Source: CAD feature listing. Evaluate the final solid. Frame: model axes, mm. Round coordinates to 2 decimals unless told otherwise and drop trailing zeros. Write each loop counter-clockwise with the first axis right and the second up, starting at its lowest first coordinate (ties: lowest second). Pieces come first, ordered by that corner, then holes. Notation, with made-up numbers: M -26,-12 L -13,-12 A26 cw -13,11 Z; hole C -31.75,63.5 d7. An arc over 180 degrees is marked long. Answer in a Markdown table with one row per item. Add a question column.
Item 1: Cut plane B-B on z = -34.75. Give the number of separate pieces and of enclosed holes in the cut face, and give its area (3 significant figures).
Item 2: Cut plane A-A on x = 276. Return loops of the section in (y, z).
Item 3: Material intervals for probe 1 along X at (y, z) = (53.75, -211.5); probe 2 along X at (y, z) = (56.25, -34.75); probe 3 along X at (y, z) = (42, -184), sorted ascending.
Item 4: Contact query for flat-ended pins moving along their axis: pin 1 (5.5 mm diameter, centred on x = 23.5, z = -34.5, fed in from +Y); pin 2 (4.5 mm diameter, centred on x = 261, z = -211.5, fed in from +Y). Output: stop coordinate, or through.
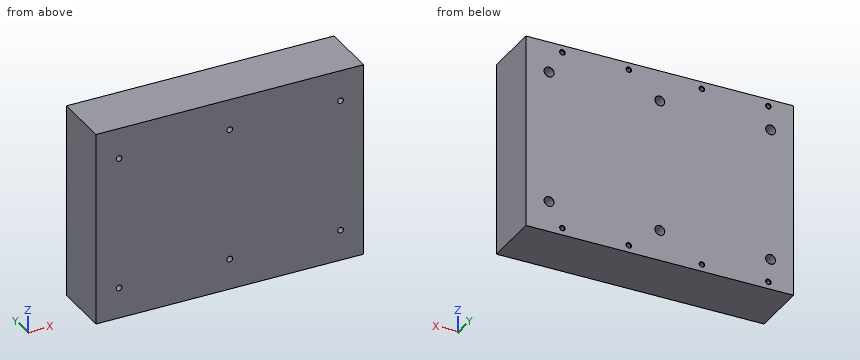
from build123d import *

# Parameters (mm, degrees)
SKETCH1_W                       = 302
SKETCH1_H                       = 219.5
BOSS_EXTRUDE1_DEPTH             = 64.4
M6X1_0_TAPPED_HOLE1_D           = 5
M6X1_0_TAPPED_HOLE1_DEPTH       = 16
M6X1_0_TAPPED_HOLE1_CSINK_D     = 6.2
M6X1_0_TAPPED_HOLE1_CSINK_ANGLE = 90
M6X1_0_TAPPED_HOLE1_TIP         = 1.502151548
CBORE_FOR_M6_SHCS1_AT_2_COUNT   = 2
CBORE_FOR_M6_SHCS1_AT_2_PITCH   = 150
CBORE_FOR_M6_SHCS1_AT_3_COUNT   = 2
CBORE_FOR_M6_SHCS1_AT_3_PITCH   = 195.256241898
CBORE_FOR_M6_SHCS1_AT_4_COUNT   = 2
CBORE_FOR_M6_SHCS1_AT_4_PITCH   = 125
CBORE_FOR_M6_SHCS1_AT_5_COUNT   = 2
CBORE_FOR_M6_SHCS1_AT_5_PITCH   = 250
CBORE_FOR_M6_SHCS1_AT_6_COUNT   = 2
CBORE_FOR_M6_SHCS1_AT_6_PITCH   = 291.547594742


with BuildPart() as part:
    # Sketch1 → Boss-Extrude1 (new body)
    with BuildSketch(Plane(origin=(0, 0, 0), x_dir=(1, 0, 0), z_dir=(0, 1, 0))):
        with Locations((151, 109.75)):
            Rectangle(SKETCH1_W, SKETCH1_H)
    extrude(amount=BOSS_EXTRUDE1_DEPTH)

    # M6x1.0 Tapped Hole1
    with Locations(Plane(origin=(0, 64.4, 0), x_dir=(1, 0, 0), z_dir=(0, 1, 0))):
        with Locations((28.5, 8), (103.5, 8), (186, 8), (261, 8), (261, 211.5), (186, 211.5), (103.5, 211.5), (28.5, 211.5)):
            CounterSinkHole(M6X1_0_TAPPED_HOLE1_D / 2, M6X1_0_TAPPED_HOLE1_CSINK_D / 2, depth=M6X1_0_TAPPED_HOLE1_DEPTH, counter_sink_angle=M6X1_0_TAPPED_HOLE1_CSINK_ANGLE)
            with Locations((0, 0, -(M6X1_0_TAPPED_HOLE1_DEPTH + M6X1_0_TAPPED_HOLE1_TIP / 2))):  # 118° drill point
                Cone(0, M6X1_0_TAPPED_HOLE1_D / 2, M6X1_0_TAPPED_HOLE1_TIP, mode=Mode.SUBTRACT)

    # Sketch5 → CBORE for M6 SHCS1 (revolve, cut)
    with BuildSketch(Plane(origin=(26, 64.4, -34.75), x_dir=(0, 0, 1), z_dir=(1, 0, 0))):
        Polygon((0, 0), (0, 64.4), (3.2, 64.4), (3.2, 20), (5.5, 20), (5.5, 0.1), (5.6, 0), align=None)
    cbore_for_m6_shcs1 = revolve(axis=Axis((26, 70.75, -34.75), (0, -1, 0)), mode=Mode.SUBTRACT)

    # CBORE for M6 SHCS1 at 2: CBORE for M6 SHCS1 ×2
    with Locations(*[(0, 0, -i * CBORE_FOR_M6_SHCS1_AT_2_PITCH) for i in range(1, CBORE_FOR_M6_SHCS1_AT_2_COUNT)]):
        add(cbore_for_m6_shcs1, mode=Mode.SUBTRACT)

    # CBORE for M6 SHCS1 at 3: CBORE for M6 SHCS1 ×2
    with Locations(*[Vector(0.6401844, 0, -0.76822128) * (i * CBORE_FOR_M6_SHCS1_AT_3_PITCH) for i in range(1, CBORE_FOR_M6_SHCS1_AT_3_COUNT)]):
        add(cbore_for_m6_shcs1, mode=Mode.SUBTRACT)

    # CBORE for M6 SHCS1 at 4: CBORE for M6 SHCS1 ×2
    with Locations(*[(i * CBORE_FOR_M6_SHCS1_AT_4_PITCH, 0, 0) for i in range(1, CBORE_FOR_M6_SHCS1_AT_4_COUNT)]):
        add(cbore_for_m6_shcs1, mode=Mode.SUBTRACT)

    # CBORE for M6 SHCS1 at 5: CBORE for M6 SHCS1 ×2
    with Locations(*[(i * CBORE_FOR_M6_SHCS1_AT_5_PITCH, 0, 0) for i in range(1, CBORE_FOR_M6_SHCS1_AT_5_COUNT)]):
        add(cbore_for_m6_shcs1, mode=Mode.SUBTRACT)

    # CBORE for M6 SHCS1 at 6: CBORE for M6 SHCS1 ×2
    with Locations(*[Vector(0.857492926, 0, -0.514495755) * (i * CBORE_FOR_M6_SHCS1_AT_6_PITCH) for i in range(1, CBORE_FOR_M6_SHCS1_AT_6_COUNT)]):
        add(cbore_for_m6_shcs1, mode=Mode.SUBTRACT)


solid = part.part
Results below:
| question | item | result |
|---|---|---|
| 1 | separate pieces | 4 |
| 1 | enclosed holes | 0 |
| 1 | area | 17,900 mm2 |
| 2 | outline | M 0,-219.5 L 64.4,-219.5 L 64.4,-190.35 L 64.3,-190.25 L 44.4,-190.25 L 44.4,-187.95 L 0,-187.95 Z; M 0,-181.55 L 44.4,-181.55 L 44.4,-179.25 L 64.3,-179.25 L 64.4,-179.15 L 64.4,-40.35 L 64.3,-40.25 L 44.4,-40.25 L 44.4,-37.95 L 0,-37.95 Z; M 0,-31.55 L 44.4,-31.55 L 44.4,-29.25 L 64.3,-29.25 L 64.4,-29.15 L 64.4,0 L 0,0 Z |
| 3 | probe 1 | 0 to 26, 31 to 101, 106 to 183.5, 188.5 to 258.5, 263.5 to 302 |
| 3 | probe 2 | 0 to 20.5, 31.5 to 145.5, 156.5 to 270.5, 281.5 to 302 |
| 3 | probe 3 | 0 to 22.89, 29.11 to 147.89, 154.11 to 272.89, 279.11 to 302 |
| 4 | pin 1 | y = 44.4 |
| 4 | pin 2 | y = 48.25 |
